Solid Edge part; units mm, degrees
sketch "Sketch1" plane through (0, 0, 0) normal (0, 0, 1) x (1, 0, 0)
  circle A0 centre (0, 0) radius 5
extrude "Protrusion1" add sketch "Sketch1" along normal blind 1.5
sketch "Sketch2" plane through (0, 0, 0) normal (0, 0, 1) x (1, 0, 0)
  line L0 (-1, 4) -> (-1, -4)
  line L1 (-1, -4) -> (1, -4)
  line L2 (1, -4) -> (1, 4)
  line L3 (1, 4) -> (-1, 4)
extrude "Protrusão_Extrudada_2" add sketch "Sketch2" along normal blind 2.3
sketch "Sketch3" plane through (0, 0, 0) normal (0, 0, 1) x (1, 0, 0)
  line L0 (-4, -1) -> (4, -1)
  line L1 (4, -1) -> (4, 1)
  line L2 (4, 1) -> (-4, 1)
  line L3 (-4, 1) -> (-4, -1)
extrude "Protrusão_Extrudada_3" add sketch "Sketch3" along normal blind 2.3
sketch "Sketch4" plane through (0, 0, 0) normal (0, 0, -1) x (-1, 0, 0)
  circle A0 centre (0, 0) radius 2.5
extrude "Protrusão_Extrudada_5" add sketch "Sketch4" along normal blind 5
fillet "Redondo_1" radius 1 1 edges at (2.5, 0, 0)
Verification items for the finished model (mm, model axes). A direction names the side the tool comes from. Round coordinates to 2 decimals unless told otherwise and drop trailing zeros. Loops run counter-clockwise (first coordinate to the right, second up) from the corner with the lowest first, then second, coordinate; pieces in that order, holes last. Notation, with made-up numbers: (34, -26) - (52, -26) arc R30 cw to (52, 0) - close; hole circle Ø1 at (-29, 35). An arc over 180 degrees is marked (long way). Write item = value, one per line.
Q1. Tool access check on faces 1 (the cylindrical face through (-1.08, 4.88, 0.74)), 2 (the cylindrical face through (0.54, 2.44, -2.97)). Record the directions out of +Z, -Z, +X, -X, +Y, -Y that give a thin tool (end or side, any length) a straight path to the whole face; none if there is none.
Here are the results:
face_1 = +Z, -Z
face_2 = -Z
Q2. Material ranges on L1, parallel to Z at x = -3.5, y = 1.75; L2, parallel to Y at x = 0.25, z = 1.75; L3, parallel to X at y = 1.75, z = -0.5, recorded low to high.
Here are the results:
L1 = 0 to 1.5
L2 = -4 to 4
L3 = -1.97 to 1.97
Q3. Sectioned sample at A-A on x = 0. Record the boundary of the cut face in (y, z).
Here are the results:
outline = (-5, 0) - (-3.5, 0) arc R1 cw to (-2.5, -1) - (-2.5, -5) - (2.5, -5) - (2.5, -1) arc R1 cw to (3.5, 0) - (5, 0) - (5, 1.5) - (4, 1.5) - (4, 2.3) - (-4, 2.3) - (-4, 1.5) - (-5, 1.5) - close
Q4. Sectioned sample at D-D on z = -0.5. Record the boundary of the cut face in (x, y).
Here are the results:
outline = circle Ø5.27 at (0, 0)
Q5. Sectioned sample at C-C on z = -1.75. Record the boundary of the cut face in (x, y).
Here are the results:
outline = circle Ø5 at (0, 0)
Q6. Depth check by flat-ended pin: pin 1 (1 mm diameter, centred on y = -0.5, z = 0, fed in from +X); pin 2 (3 mm diameter, centred on y = -1, z = -4, fed in from +X); pin 3 (0.9 mm diameter, centred on x = -2.5, z = 2, fed in from +Y); pin 4 (0.6 mm diameter, centred on y = -0.5, z = 2, fed in from +X). Enter the tip coordinate at first touch or a pass-through.
Here are the results:
pin_1 = 5
pin_2 = 2.5
pin_3 = 1
pin_4 = 4
